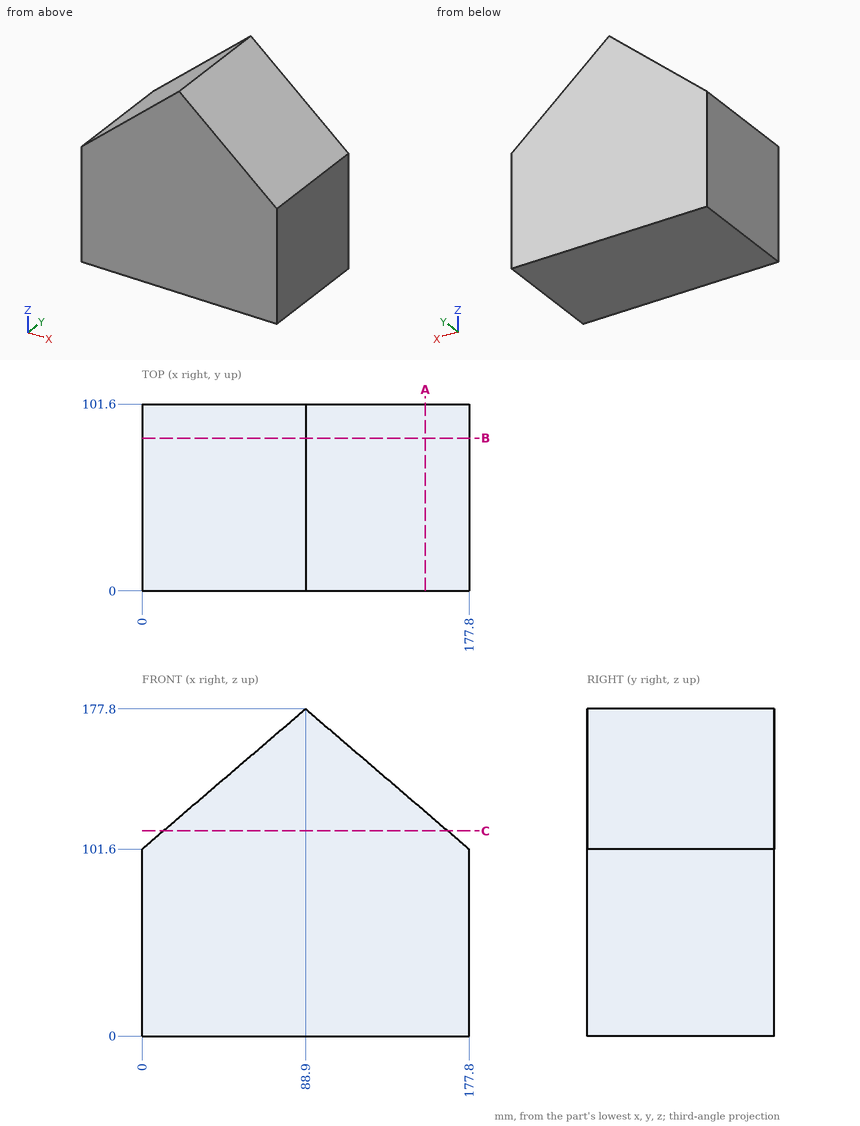
Drawing for the job (mm, zero at the part's lowest x, y, z). Coordinates: 2 decimals unless noted, no trailing zeros. Order: outer loops, then holes, each group sorted by start corner. A loop starts at its lowest first (then second) coordinate and runs counter-clockwise, first axis right, second up.
Item 1: Band-saw the part on C-C on z = 111.5. List the corners of the cut face in (x, y).
Check sheet entries:
outline: (11.55, 0) - (166.25, 0) - (166.25, 101.6) - (11.55, 101.6) - close
Item 2: Drill centre lines: L1, parallel to Z at x = 51.5, y = 68; L2, parallel to Z at x = 52.5, y = 40; L3, parallel to X at y = 61, z = 134.5. Where is each one in solid material? Low to high.
Check sheet entries:
L1: z = 0 to 145.74
L2: z = 0 to 146.6
L3: x = 38.38 to 139.42
Item 3: Pin check, flat tips, straight feed: pin 1 Ø2 at (x, y) = (83, 38.5) entering from -Z; pin 2 Ø1.5 at (x, y) = (136.5, 31.5) entering from +Z; pin 3 Ø4 at (y, z) = (71.5, 155) entering from +X; pin 4 Ø1 at (x, y) = (59.5, 62.5) entering from +Z. Stop position of each tip, or through.
Check sheet entries:
pin 1: stops at z = 0
pin 2: stops at z = 137.64
pin 3: stops at x = 117.83
pin 4: stops at z = 153.03
Item 4: Band-saw the part on A-A on x = 154. List the corners of the cut face in (y, z).
Check sheet entries:
outline: (0, 0) - (101.6, 0) - (101.6, 122) - (0, 122) - close
Item 5: Band-saw the part on B-B on y = 83. List the corners of the cut face in (x, z).
Check sheet entries:
outline: (0, 0) - (177.8, 0) - (177.8, 101.6) - (88.9, 177.8) - (0, 101.6) - close
